```python
from build123d import *

# Parameters (mm, degrees)
SKETCH1_W           = 24
SKETCH1_H           = 20
SKETCH1_R           = 1.6
BOSS_EXTRUDE1_DEPTH = 18
BOSS_EXTRUDE2_DEPTH = 6
SKETCH3_R           = 2.5
BOSS_EXTRUDE3_DEPTH = 7
FILLET1_R           = 1
CHAMFER1_SIZE       = 2.5


with BuildPart() as part:
    # Sketch1 → Boss-Extrude1 (new body)
    with BuildSketch(Plane.XY):
        Rectangle(SKETCH1_W, SKETCH1_H)
        with Locations((-5, 5)):
            Circle(SKETCH1_R, mode=Mode.SUBTRACT)
        with Locations((-5, -5)):
            Circle(SKETCH1_R, mode=Mode.SUBTRACT)
    extrude(amount=BOSS_EXTRUDE1_DEPTH)

    # Sketch2 → Boss-Extrude2 (add)
    with BuildSketch(Plane(origin=(12, 0, 0), x_dir=(0, 0, -1), z_dir=(1, 0, 0))):
        Polygon((-18, -10), (-18, 10), (-43, 2), (-88, 2), (-88, -10), align=None)
    extrude(amount=-BOSS_EXTRUDE2_DEPTH)

    # Sketch3 → Boss-Extrude3 (add)
    with BuildSketch(Plane(origin=(0, -7.5, 0), x_dir=(-1, 0, 0), z_dir=(0, -1, 0))):
        with Locations((-6, -83)):
            Circle(SKETCH3_R)
        with Locations((-6, -65)):
            Circle(SKETCH3_R)
    extrude(amount=-BOSS_EXTRUDE3_DEPTH)

    # Fillet1
    fillet1_edges = [part.edges().sort_by_distance(p)[0] for p in [
        (6, -4, 80.5),
        (6, -4, 85.5),
        (6, -4, 62.5),
        (6, -4, 67.5),
    ]]
    fillet(fillet1_edges, radius=FILLET1_R)

    # Chamfer1
    chamfer1_edges = [part.edges().sort_by_distance(p)[0] for p in [
        (6, -0.5, 83),
    ]]
    chamfer(chamfer1_edges, length=CHAMFER1_SIZE - 0.0001)  # a hair under: the kernel refuses the full size
    chamfer1_2_edges = [part.edges().sort_by_distance(p)[0] for p in [
        (6, -7.5, 83),
    ]]
    chamfer(chamfer1_2_edges, length=CHAMFER1_SIZE - 0.0001)  # a hair under: the kernel refuses the full size
    chamfer1_3_edges = [part.edges().sort_by_distance(p)[0] for p in [
        (6, -0.5, 65),
    ]]
    chamfer(chamfer1_3_edges, length=CHAMFER1_SIZE - 0.0001)  # a hair under: the kernel refuses the full size
    chamfer1_4_edges = [part.edges().sort_by_distance(p)[0] for p in [
        (6, -7.5, 65),
    ]]
    chamfer(chamfer1_4_edges, length=CHAMFER1_SIZE - 0.0001)  # a hair under: the kernel refuses the full size


solid = part.part
```
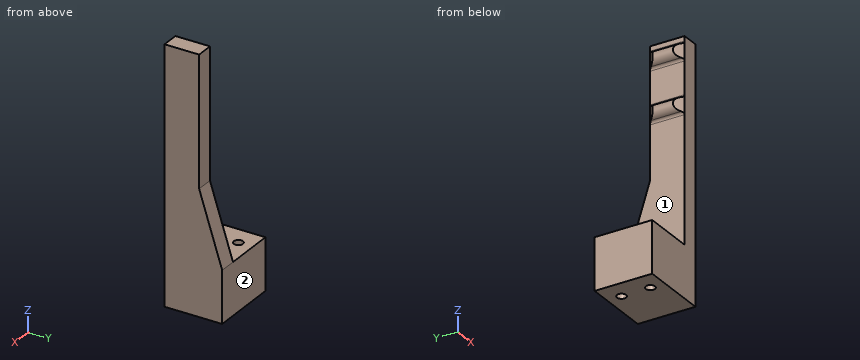
Can you work these out from the model? Positions are in its coordinate system, mm. Face numbers are marked on the shaded views. A direction names the side the tool comes from. Give positions to 0.01 mm unless a question says otherwise; leave off trailing zeros. Write each loop counter-clockwise with the first axis right and the second up, starting at its lowest first coordinate (ties: lowest second). Pieces come first, ordered by that corner, then holes. Notation, with made-up numbers: (61.5, -36) -> (85.5, -36) arc R28 ccw to (85.5, -11) -> close; hole circle Ø5 at (77.25, 71.25). An arc over 180 degrees is marked (long way). One line per item, written item: value.
Q1. Imagine slicing it at B-B on y = -5. Please give me the cut outline in (x, z), and give its area (3 significant figures).
Results found:
outline: (-12, 0) -> (-6.6, 0) -> (-6.6, 18) -> (-12, 18) -> close; (-3.4, 0) -> (12, 0) -> (12, 88) -> (6, 88) -> (6, 86.35) arc R1 cw to (5.29, 85.4) arc R2.5 ccw to (5.29, 80.6) arc R1 cw to (6, 79.65) -> (6, 68.35) arc R1 cw to (5.29, 67.4) arc R2.5 ccw to (5.29, 62.6) arc R1 cw to (6, 61.65) -> (6, 18) -> (-3.4, 18) -> close
area: 815 mm^2
Q2. Which directions (+Z, -Z, +X, -X, +Y, -Y) give clear straight access to the entire face, cutting with the end or side of a thin tool? Please do the marked faces 1 and 2.
Results found:
face 1: -X, +Y, -Y
face 2: +Z, -Z, +X, -X, +Y
Q3. Please list where these lines run through material, in increasing order: line 1 (Y direction, x = -5, z = 11.75); line 2 (Z direction, x = 4.25, y = -1); line 3 (Z direction, x = -2.5, y = -2). Write a range as [from, to].
Results found:
line 1: y = [-10, -6.6], [-3.4, 3.4], [6.6, 10]
line 2: z = [0, 18], [63.21, 66.79], [81.21, 84.79]
line 3: z = [0, 18]
Q4. Imagine slicing it at A-A on x = -5. Please give me the cut outline in (y, z), and give its area (3 significant figures).
Results found:
outline: (-10, 0) -> (-6.6, 0) -> (-6.6, 18) -> (-10, 18) -> close; (-3.4, 0) -> (3.4, 0) -> (3.4, 18) -> (-3.4, 18) -> close; (6.6, 0) -> (10, 0) -> (10, 18) -> (6.6, 18) -> close
area: 245 mm^2
Q5. For P1, Ø10, axis at y = 4, z = 25, coming from the -X side; P2, Ø1, axis at x = -8, y = -4, coming from the +Z side; P3, Ø1.8, axis at x = 9, z = 55.5, coming from the +Y side, each with a flat end and sliding along its axis, tell me the tip position at first contact or that it passes through.
Results found:
P1: stops at x = 6
P2: stops at z = 18
P3: stops at y = 2
Q6. Imagine slicing it at C-C on z = 8. Please give me the cut outline in (x, y), and give its area (3 significant figures).
Results found:
outline: (-12, -10) -> (12, -10) -> (12, 10) -> (-12, 10) -> close; hole circle Ø3.2 at (-5, -5); hole circle Ø3.2 at (-5, 5)
area: 464 mm^2
Q7. Imagine slicing it at D-D on x = 8.25. Please give me the cut outline in (y, z).
Results found:
outline: (-10, 0) -> (10, 0) -> (10, 18) -> (2, 43) -> (2, 88) -> (-10, 88) -> close
